from build123d import *

# Parameters (mm, degrees)
SKETCH1_R           = 7
SKETCH1_R_2         = 2.5
BOSS_EXTRUDE1_DEPTH = 22.5
SKETCH2_W           = 21.9
SKETCH2_H           = 63.25
CUT_EXTRUDE1_DEPTH  = 136.25346576
SKETCH3_R           = 7.5
CUT_EXTRUDE2_DEPTH  = 1
CUT_EXTRUDE3_START  = -1
SKETCH4_R           = 7.5
CUT_EXTRUDE3_DEPTH  = 1
SKETCH5_W           = 9.8
SKETCH5_H           = 70
CUT_EXTRUDE4_DEPTH  = 136.25346576
CUT_EXTRUDE5_DEPTH  = 135.872393395
CUT_EXTRUDE6_REACH  = 148.858
SKETCH8_W           = 46.5
SKETCH8_H           = 1.95
SKETCH9_W           = 50.8
SKETCH9_H           = 25.4
BOSS_EXTRUDE2_DEPTH = 5
FILLET1_R           = 10
CHAMFER1_SIZE       = 5
CHAMFER2_SIZE       = 2


# Some blends are built 0.0001 mm under size
with BuildPart() as part:
    # Sketch1 → Boss-Extrude1 (new, symmetric)
    with BuildSketch(Plane.XY):
        with BuildLine():
            Line((-23.25, 0), (-23.25, 125))
            Line((-23.25, 125), (23.25, 125))
            Line((23.25, 125), (23.25, 0))
            ThreePointArc((23.25, 0), (0, -23.25), (-23.25, 0))
        make_face()
        with Locations(Location((0, 0, 0), (0, 0, 180))):
            Circle(SKETCH1_R, mode=Mode.SUBTRACT)
        with Locations(Location((-11.25, 110, 0), (0, 0, 180))):
            Circle(SKETCH1_R_2, mode=Mode.SUBTRACT)
        with Locations(Location((11.25, 110, 0), (0, 0, 180))):
            Circle(SKETCH1_R_2, mode=Mode.SUBTRACT)
        with Locations(Location((11.25, 75, 0), (0, 0, 180))):
            Circle(SKETCH1_R_2, mode=Mode.SUBTRACT)
        with Locations(Location((-11.25, 75, 0), (0, 0, 180))):
            Circle(SKETCH1_R_2, mode=Mode.SUBTRACT)
    extrude(amount=BOSS_EXTRUDE1_DEPTH, both=True)

    # Sketch2 → Cut-Extrude1 (cut, through all)
    with BuildSketch(Plane(origin=(23.25, 0, 0), x_dir=(0, 0, -1), z_dir=(1, 0, 0))):
        with Locations((0, 8.375)):
            Rectangle(SKETCH2_W, SKETCH2_H)
    extrude(amount=-CUT_EXTRUDE1_DEPTH, mode=Mode.SUBTRACT)

    # Sketch3 → Cut-Extrude2 (cut)
    with BuildSketch(Plane.XY.offset(22.5)):
        Circle(SKETCH3_R)
    extrude(amount=-CUT_EXTRUDE2_DEPTH, mode=Mode.SUBTRACT)

    # Sketch4 → Cut-Extrude3 (cut)
    with BuildSketch(Plane(origin=(0, 0, -22.5), x_dir=(-1, 0, 0), z_dir=(0, 0, -1)).offset(CUT_EXTRUDE3_START)):
        with Locations(Location((0, 0, 0), (0, 0, 180))):
            Circle(SKETCH4_R)
    extrude(amount=CUT_EXTRUDE3_DEPTH, mode=Mode.SUBTRACT)

    # Sketch5 → Cut-Extrude4 (cut, through all)
    with BuildSketch(Plane(origin=(23.25, 0, 0), x_dir=(0, 0, -1), z_dir=(1, 0, 0))):
        with Locations((-17.6, 90)):
            Rectangle(SKETCH5_W, SKETCH5_H)
        with Locations((17.6, 90)):
            Rectangle(SKETCH5_W, SKETCH5_H)
    extrude(amount=-CUT_EXTRUDE4_DEPTH, mode=Mode.SUBTRACT)

    # Sketch6 → Cut-Extrude5 (cut, through all)
    with BuildSketch(Plane.XY.offset(22.5)):
        with BuildLine():
            Line((-18.25, 0), (-18.25, 55))
            Line((-18.25, 55), (-23.25, 55))
            Line((-23.25, 55), (-23.25, -23.25))
            Line((-23.25, -23.25), (23.25, -23.25))
            Line((23.25, -23.25), (23.25, 55))
            Line((23.25, 55), (18.25, 55))
            Line((18.25, 55), (18.25, 0))
            ThreePointArc((18.25, 0), (0, -18.25), (-18.25, 0))
        make_face()
    extrude(amount=-CUT_EXTRUDE5_DEPTH, mode=Mode.SUBTRACT)

    # Cut-Extrude6: up to this face of the body (flat: up to its plane)
    cut_extrude6_end = Plane(part.part.faces().sort_by_distance((0, 55, -17.6))[0])
    # Sketch8 → Cut-Extrude6 (cut, up to the picked face)
    with BuildSketch(Plane(origin=(0, 125, 0), x_dir=(1, 0, 0), z_dir=(0, 1, 0)), mode=Mode.PRIVATE) as cut_extrude6_sk1:
        with Locations((0, 11.725)):
            Rectangle(SKETCH8_W, SKETCH8_H)
    cut_extrude6_tool1 = split(extrude(cut_extrude6_sk1.sketch, amount=-CUT_EXTRUDE6_REACH, mode=Mode.PRIVATE), bisect_by=cut_extrude6_end, keep=Keep.BOTH, mode=Mode.PRIVATE)
    # Sketch8 → Cut-Extrude6 (cut, up to the picked face)
    with BuildSketch(Plane(origin=(0, 125, 0), x_dir=(1, 0, 0), z_dir=(0, 1, 0)), mode=Mode.PRIVATE) as cut_extrude6_sk2:
        with Locations((0, -11.725)):
            Rectangle(SKETCH8_W, SKETCH8_H)
    cut_extrude6_tool2 = split(extrude(cut_extrude6_sk2.sketch, amount=-CUT_EXTRUDE6_REACH, mode=Mode.PRIVATE), bisect_by=cut_extrude6_end, keep=Keep.BOTH, mode=Mode.PRIVATE)
    add(cut_extrude6_tool1.solids().sort_by(Axis((0, 125, -11.725), (0, -1, 0)))[0], mode=Mode.SUBTRACT)
    add(cut_extrude6_tool2.solids().sort_by(Axis((0, 125, 11.725), (0, -1, 0)))[0], mode=Mode.SUBTRACT)

    # Sketch9 → Boss-Extrude2 (add)
    with BuildSketch(Plane(origin=(0, 55, 0), x_dir=(1, 0, 0), z_dir=(0, 1, 0))):
        Rectangle(SKETCH9_W, SKETCH9_H)
    extrude(amount=-BOSS_EXTRUDE2_DEPTH)

    # Fillet1
    fillet1_edges = [part.edges().sort_by_distance(p)[0] for p in [
        (18.25, 40, 0),
        (-18.25, 40, 0),
    ]]
    fillet(fillet1_edges, radius=FILLET1_R - 0.0001)  # a hair under: the kernel refuses the full size

    # Chamfer1
    chamfer1_edges = [part.edges().sort_by_distance(p)[0] for p in [
        (-25.4, 50, 0),
        (25.4, 50, 0),
    ]]
    chamfer(chamfer1_edges, length=CHAMFER1_SIZE - 0.0001)  # a hair under: the kernel refuses the full size

    # Chamfer2
    # the kernel refuses this chamfer: 2 mm, written as the material it adds along each edge
    with BuildSketch(Plane(origin=(8.2501, 40, -10.95), x_dir=(0, -0.9996219169112968, -0.02749587661058651), z_dir=(-1, 0, 0))) as chamfer2_piece_1:
        Polygon((CHAMFER2_SIZE * 0.999621916911, CHAMFER2_SIZE * 0.0274958766106), (-CHAMFER2_SIZE * 0.0274958766106, CHAMFER2_SIZE * 0.999621916911), (0, 0), align=None)
    extrude(amount=16.5002)
    with BuildSketch(Plane(origin=(8.2501, 40, 10.95), x_dir=(0, -0.9996219169112968, 0.02749587661058651), z_dir=(-1, 0, 0))) as chamfer2_piece_2:
        Polygon((CHAMFER2_SIZE * 0.999621916911, -CHAMFER2_SIZE * 0.0274958766106), (-CHAMFER2_SIZE * 0.0274958766106, -CHAMFER2_SIZE * 0.999621916911), (0, 0), align=None)
    extrude(amount=16.5002)
    with BuildSketch(Plane(origin=(8.2501, 49.9999, 10.95), x_dir=(0, -1, 0), z_dir=(-1, 0, 0))) as chamfer2_piece_3_section:
        Polygon((9.9999 + CHAMFER2_SIZE, 0), (9.9999, -CHAMFER2_SIZE), (9.9999, 0), align=None)
    chamfer2_piece_3 = revolve(axis=Axis((8.2501, 49.9999, 10.95), (0, 0, 1)), revolution_arc=119.48144917, mode=Mode.PRIVATE)
    chamfer2_piece_3 = split(chamfer2_piece_3, bisect_by=Plane(origin=(18.25, 39.233435125, 10.852733076), z_dir=(-1, 0, 0)), keep=Keep.TOP, mode=Mode.PRIVATE)
    chamfer2_piece_3 = split(chamfer2_piece_3, bisect_by=Plane(origin=(10.698789492, 50, 10.852733076), z_dir=(0, -1, 0)), keep=Keep.TOP, mode=Mode.PRIVATE)
    add(chamfer2_piece_3)
    with BuildSketch(Plane(origin=(8.2501, 49.9999, -10.95), x_dir=(0, -1, 0), z_dir=(-1, 0, 0))) as chamfer2_piece_4_section:
        Polygon((9.9999 + CHAMFER2_SIZE, 0), (9.9999, CHAMFER2_SIZE), (9.9999, 0), align=None)
    chamfer2_piece_4 = revolve(axis=Axis((8.2501, 49.9999, -10.95), (0, 0, 1)), revolution_arc=119.48144917, mode=Mode.PRIVATE)
    chamfer2_piece_4 = split(chamfer2_piece_4, bisect_by=Plane(origin=(18.25, 39.233435125, -10.852733076), z_dir=(-1, 0, 0)), keep=Keep.TOP, mode=Mode.PRIVATE)
    chamfer2_piece_4 = split(chamfer2_piece_4, bisect_by=Plane(origin=(10.698789492, 50, -10.852733076), z_dir=(0, -1, 0)), keep=Keep.TOP, mode=Mode.PRIVATE)
    add(chamfer2_piece_4)
    with BuildSketch(Plane(origin=(-8.2501, 49.9999, -10.95), x_dir=(0, -1, 0), z_dir=(1, 0, 0))) as chamfer2_piece_5_section:
        Polygon((9.9999 + CHAMFER2_SIZE, 0), (9.9999, -CHAMFER2_SIZE), (9.9999, 0), align=None)
    chamfer2_piece_5 = revolve(axis=Axis((-8.2501, 49.9999, -10.95), (0, 0, -1)), revolution_arc=119.48144917, mode=Mode.PRIVATE)
    chamfer2_piece_5 = split(chamfer2_piece_5, bisect_by=Plane(origin=(-10.698789492, 50, -10.852733076), z_dir=(0, -1, 0)), keep=Keep.TOP, mode=Mode.PRIVATE)
    chamfer2_piece_5 = split(chamfer2_piece_5, bisect_by=Plane(origin=(-18.25, 39.233435125, -10.852733076), z_dir=(1, 0, 0)), keep=Keep.TOP, mode=Mode.PRIVATE)
    add(chamfer2_piece_5)
    with BuildSketch(Plane(origin=(-8.2501, 49.9999, 10.95), x_dir=(0, -1, 0), z_dir=(1, 0, 0))) as chamfer2_piece_6_section:
        Polygon((9.9999 + CHAMFER2_SIZE, 0), (9.9999, CHAMFER2_SIZE), (9.9999, 0), align=None)
    chamfer2_piece_6 = revolve(axis=Axis((-8.2501, 49.9999, 10.95), (0, 0, -1)), revolution_arc=119.48144917, mode=Mode.PRIVATE)
    chamfer2_piece_6 = split(chamfer2_piece_6, bisect_by=Plane(origin=(-10.698789492, 50, 10.852733076), z_dir=(0, -1, 0)), keep=Keep.TOP, mode=Mode.PRIVATE)
    chamfer2_piece_6 = split(chamfer2_piece_6, bisect_by=Plane(origin=(-18.25, 39.233435125, 10.852733076), z_dir=(1, 0, 0)), keep=Keep.TOP, mode=Mode.PRIVATE)
    add(chamfer2_piece_6)


solid = part.part
Build history of the part. All positions in model axes, mm. A direction names the side the tool comes from. Coordinates: 2 decimals unless noted, no trailing zeros. Order: outer loops, then holes, each group sorted by start corner. A loop starts at its lowest first (then second) coordinate and runs counter-clockwise, first axis right, second up. Notation, with made-up numbers: (62, 19) -> (90, 19) arc R28 ccw to (90, 50) -> close; hole circle Ø1 at (-12, 88). An arc over 180 degrees is marked (long way). One line per item, written item: value.
(1) Drop flat-ended pins along their axis: pin 1 Ø1.5 at (x, y) = (23, 52.5) entering from -Z; pin 2 Ø6 at (x, z) = (-0.5, 2) entering from -Y; pin 3 Ø4 at (x, y) = (-18, 70) entering from +Z; pin 4 Ø7.5 at (x, y) = (0.5, -0.5) entering from +Z. Give the stop position or say it passes through.
Checked values:
pin 1: z = -12.7
pin 2: y = 40
pin 3: z = 10.75
pin 4: through
(2) Mould opens along Z. For faces 1 (the flat face through (0, 12, 10.95)), 2 (the flat face through (-21, 53, 12.7)), 3 (the flat face through (4, 55, -12)) say: pulls with the +Z half, pulls with the -Z half, needs draft (parallel to the pull), parting line crosses it, or undercut.
Checked values:
face 1: undercut
face 2: pulls with the +Z half
face 3: needs draft
(3) Slice it at A-A, the plane z = -1. Count the separate pieces of the cut face and the enclosed holes in it, plus the area to 3 significant figures.
Checked values:
separate pieces: 1
enclosed holes: 4
area: 3,730 mm2
(4) Probe line 1 (Z direction, x = 5.5, y = 30.5); line 2 (Y direction, x = 11.25, z = 5); line 3 (Y direction, x = 11, z = 5). List the from-to ranges inside material, lowest first. Write a range as [from, to].
Checked values:
line 1: [-22.5, -10.95], [10.95, 22.5]
line 2: [40.46, 72.5], [77.5, 107.5], [112.5, 125]
line 3: [40.39, 72.51], [77.49, 107.51], [112.49, 125]
(5) Slice it at B-B, the plane y = 110. List the corners of the cut face in (x, z).
Checked values:
outline: (-23.25, -10.75) -> (-13.75, -10.75) -> (-13.75, 10.75) -> (-23.25, 10.75) -> close; (-8.75, -10.75) -> (8.75, -10.75) -> (8.75, 10.75) -> (-8.75, 10.75) -> close; (13.75, -10.75) -> (23.25, -10.75) -> (23.25, 10.75) -> (13.75, 10.75) -> close
(6) Slice it at D-D, the plane y = 32.5. List the corners of the cut face in (x, z).
Checked values:
outline: (-18.25, -22.5) -> (18.25, -22.5) -> (18.25, -10.95) -> (-18.25, -10.95) -> close; (-18.25, 10.95) -> (18.25, 10.95) -> (18.25, 22.5) -> (-18.25, 22.5) -> close
(7) Tool access for faces 4 (the flat face through (0, 90, 10.75)), 5 (the cylindrical face through (-7.493, 0.33, 22.007)), 6 (the flat face through (-21, 53, -12.7)): list every direction of +Z, -Z, +X, -X, +Y, -Y with a clear straight run to the whole face (end or side of a thin tool).
Checked values:
face 4: +Z, +X, -X, +Y
face 5: +Z
face 6: -Z, -X, +Y, -Y
